```python
from build123d import *
from OCP.BRepFilletAPI import BRepFilletAPI_MakeChamfer

# Parameters (mm, degrees)
SKETCH1_R               = 4.765
BOSS_EXTRUDE1_DEPTH     = 9.5
CHAMFER1_SIZE           = 7.62
CHAMFER1_SIZE2          = 2.54
CHAMFER2_SIZE           = 2.54
CHAMFER2_SIZE2          = 7.62
CUT_EXTRUDE1_DEPTH      = 32.662585176
CUT_EXTRUDE1_DEPTH_BACK = 32.662585176
SKETCH2_W               = 9.53
SKETCH2_H               = 8.9
CUT_EXTRUDE2_DEPTH      = 32.662585176
CUT_EXTRUDE2_DEPTH_BACK = 32.662585176
CUT_EXTRUDE3_DEPTH      = 32.662585236
CUT_EXTRUDE3_DEPTH_BACK = 32.662585236
SKETCH4_R               = 1.59


with BuildPart() as part:
    # Sketch1 → Boss-Extrude1 (new, symmetric)
    with BuildSketch(Plane.XY):
        with BuildLine():
            Line((0, 9.77), (-22.23, 9.77))
            Line((-22.23, 9.77), (-22.23, 4.77))
            Line((-22.23, 4.77), (-9.711509246, -1.067468107))
            ThreePointArc((-9.711509246, -1.067468107), (-5.877874817, -7.804068659), (1.655323868, -9.628748771))
            Line((1.655323868, -9.628748771), (28.58, -5))
            Line((28.58, -5), (28.58, 0))
            Line((28.58, 0), (9.77, 0))
            ThreePointArc((9.77, 0), (6.908433252, 6.908433252), (0, 9.77))
        make_face()
        Circle(SKETCH1_R, mode=Mode.SUBTRACT)
    extrude(amount=BOSS_EXTRUDE1_DEPTH, both=True)

    # Chamfer1
    chamfer1_edges = [part.edges().sort_by_distance(p)[0] for p in [
        (-22.23, 7.27, -9.5),
        (28.58, -2.5, -9.5),
    ]]
    chamfer1_side = [part.faces().sort_by_distance(p)[0] for p in [
        (-11.115, 9.225622585, -9.5),
    ]]
    chamfer(chamfer1_edges, length=CHAMFER1_SIZE, length2=CHAMFER1_SIZE2, reference=chamfer1_side[0])

    # Chamfer2: one chamfer whose edges measure the first distance from different faces: ONE call of the kernel's chamfer builder (chamfer() names one face for all edges)
    chamfer2_edges_1 = [part.edges().sort_by_distance(p)[0] for p in [
        (-22.23, 7.27, 9.5),
    ]]
    chamfer2_side_1 = [part.faces().sort_by_distance(p)[0] for p in [
        (-22.23, 7.27, 1.27),
    ]]
    chamfer2_edges_2 = [part.edges().sort_by_distance(p)[0] for p in [
        (28.58, -2.5, 9.5),
    ]]
    chamfer2_side_2 = [part.faces().sort_by_distance(p)[0] for p in [
        (28.58, -2.5, 1.27),
    ]]
    chamfer2 = BRepFilletAPI_MakeChamfer(part.part.solid().wrapped)
    for e in chamfer2_edges_1:
        chamfer2.Add(CHAMFER2_SIZE, CHAMFER2_SIZE2, e.wrapped, chamfer2_side_1[0].wrapped)  # the first distance lies on this face
    for e in chamfer2_edges_2:
        chamfer2.Add(CHAMFER2_SIZE, CHAMFER2_SIZE2, e.wrapped, chamfer2_side_2[0].wrapped)  # the first distance lies on this face
    add(Compound.cast(chamfer2.Shape()), mode=Mode.REPLACE)

    # Sketch2 → Cut-Extrude1 (cut, two sides: drawn at the far end of the back side and taken through both)
    with BuildSketch(Plane(origin=(0, 0, 0), x_dir=(1, 0, 0), z_dir=(0, 1, 0)).offset(-CUT_EXTRUDE1_DEPTH_BACK)):
        with Locations((-17.465, 0)):
            Rectangle(SKETCH2_W, SKETCH2_H)
        with Locations((23.815, 0)):
            Rectangle(SKETCH2_W, SKETCH2_H)
    extrude(amount=CUT_EXTRUDE1_DEPTH + CUT_EXTRUDE1_DEPTH_BACK, mode=Mode.SUBTRACT)

    # Sketch3 → Cut-Extrude2 (cut, two sides: drawn at the far end of the back side and taken through both)
    with BuildSketch(Plane(origin=(0, 0, 0), x_dir=(1, 0, 0), z_dir=(0, 1, 0)).offset(-CUT_EXTRUDE2_DEPTH_BACK)):
        with BuildLine():
            Line((-3.81, 5.08), (6.35, 5.08))
            ThreePointArc((6.35, 5.08), (11.43, 0), (6.35, -5.08))
            Line((6.35, -5.08), (-3.81, -5.08))
            ThreePointArc((-3.81, -5.08), (-8.89, 0), (-3.81, 5.08))
        make_face()
    extrude(amount=CUT_EXTRUDE2_DEPTH + CUT_EXTRUDE2_DEPTH_BACK, mode=Mode.SUBTRACT)

    # Sketch4 → Cut-Extrude3 (cut, two sides: drawn at the far end of the back side and taken through both)
    with BuildSketch(Plane.XY.offset(-CUT_EXTRUDE3_DEPTH_BACK)):
        with Locations((-19.69, 7.23)):
            Circle(SKETCH4_R)
        with Locations((26.04, -2.54)):
            Circle(SKETCH4_R)
    extrude(amount=CUT_EXTRUDE3_DEPTH + CUT_EXTRUDE3_DEPTH_BACK, mode=Mode.SUBTRACT)


solid = part.part
```
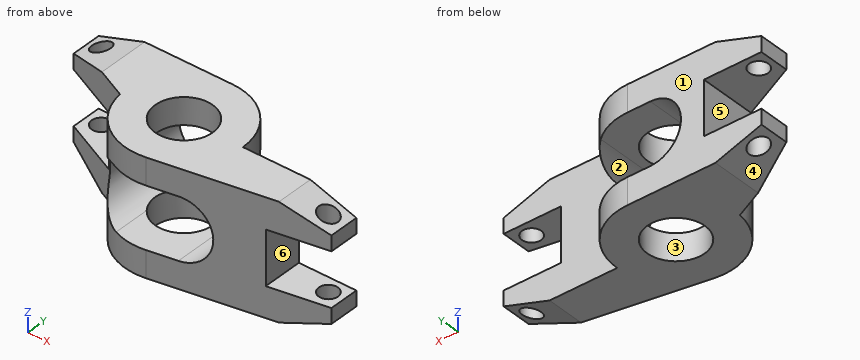
Part model, mm, in its own coordinate system. Face numbers are marked on the shaded views. A direction names the side the tool comes from. Coordinates: 2 decimals unless noted, no trailing zeros. Order: outer loops, then holes, each group sorted by start corner. A loop starts at its lowest first (then second) coordinate and runs counter-clockwise, first axis right, second up. Notation, with made-up numbers: (-31, 38.25) - (21, 38.25) arc R24 cw to (21, 48.25) - close; hole circle Ø8 at (-36.75, 13). An arc over 180 degrees is marked (long way). Return JSON: item names as keys, results as strings. Group by question number.
Item 1: Pin check, flat tips, straight feed: pin 1 (4.5 mm diameter, centred on x = -17, y = 3.5, fed in from +Z); pin 2 (3.5 mm diameter, centred on x = 26.04, y = -2.54, fed in from +Z); pin 3 (10 mm diameter, centred on x = 3.5, z = 7.5, fed in from +Y); pin 4 (9.5 mm diameter, centred on x = 16.5, z = -2, fed in from +Y). Stop position of each tip, or through.
Item 2: Drill centre lines: probe 1 along Z at (x, y) = (-0.5, -8); probe 2 along Y at (x, z) = (0.5, -8); probe 3 along Y at (x, z) = (26, 5.25). Where is each one in solid material? Low to high. Write a range as from..to.
Item 3: Which spindle directions (+Z, -Z, +X, -X, +Y, -Y) get a long thin tool onto all of the face, cutting with end or side? Do the marked faces 4, 5 and 6. Say none if no direction does.
Item 4: Cut at A-A (x = -14). List the corners of the cut face in (y, z).
Item 5: Cut at B-B (z = 1.5). List the corners of the cut face in (x, y), plus the area to 3 significant figures.
Item 6: Pull direction Y, two halves, no side cores. Call the marked faces 1, 2 and 3: pulls with the +Y half, pulls with the -Y half, needs draft (parallel to the pull), parting line crosses it, or undercut.
Item 7: Cut at C-C (x = -19.69). List the corners of the cut face in (y, z), plus the area to 3 significant figures.
Item 8: Cut at D-D (y = -5.75). List the corners of the cut face in (x, z).
Check values:
{
 "1": {"pin 1": "stops at z = 9.45", "pin 2": "stops at z = 8.39", "pin 3": "stops at y = 9.77", "pin 4": "stops at y = 0"},
 "2": {"probe 1": "z = -9.5..-5.08, 5.08..9.5", "probe 2": "y = -9.76..-4.74, 4.74..9.76", "probe 3": "y = -5.44..-4.13, -0.95..0"},
 "3": {"face 4": "-Z, -X, +Y, -Y", "face 5": "-X, +Y, -Y", "face 6": "+X, +Y, -Y"},
 "4": {"outline": "(0.93, -9.5) - (9.77, -9.5) - (9.77, -4.45) - (0.93, -4.45) - close; (0.93, 4.45) - (9.77, 4.45) - (9.77, 9.5) - (0.93, 9.5) - close"},
 "5": {"outline": "(-12.7, 0.33) - (-9.71, -1.07) arc R9.77 ccw to (-8.66, -4.52) - (-8.66, 9.77) - (-12.7, 9.77) - close; (11.2, -7.99) - (19.05, -6.64) - (19.05, 0) - (11.2, 0) - close", "area": "101 mm2"},
 "6": {"face 1": "pulls with the +Y half", "face 2": "needs draft", "face 3": "undercut"},
 "7": {"outline": "(3.59, -7.81) - (5.64, -7.81) - (5.64, -4.45) - (3.59, -4.45) - close; (3.59, 4.45) - (5.64, 4.45) - (5.64, 7.81) - (3.59, 7.81) - close; (8.82, -7.81) - (9.77, -7.81) - (9.77, -4.45) - (8.82, -4.45) - close; (8.82, 4.45) - (9.77, 4.45) - (9.77, 7.81) - (8.82, 7.81) - close", "area": "20.2 mm2"},
 "8": {"outline": "(-7.9, -9.5) - (20.96, -9.5) - (24.22, -8.41) - (24.22, -4.45) - (19.05, -4.45) - (19.05, 4.45) - (24.22, 4.45) - (24.22, 8.41) - (20.96, 9.5) - (-7.9, 9.5) - (-7.9, 3.01) arc R5.08 cw to (-3.81, 5.08) - (6.35, 5.08) arc R5.08 cw to (6.35, -5.08) - (-3.81, -5.08) arc R5.08 cw to (-7.9, -3.01) - close"}
}
